Can you work these out from the model? Positions are in its coordinate system, mm. Face numbers are marked on the shaded views. A direction names the side the tool comes from. Round coordinates to 2 decimals unless told otherwise and drop trailing zeros. Write each loop counter-clockwise with the first axis right and the second up, starting at its lowest first coordinate (ties: lowest second). Pieces come first, ordered by that corner, then holes. Notation, with made-up numbers: M -9,6.25 L 40,6.25 A25 ccw 40,44.25 Z; hole C 9.25,-25 d1. An arc over 180 degrees is marked long. Use one line per item in the form item = value. Start each with the question number.
```python
from build123d import *

# Parameters (mm, degrees)
SKETCH1_W           = 20.1
SKETCH1_H           = 20.1
BOSS_EXTRUDE1_DEPTH = 40
SKETCH1_3_R         = 5.1
BOSS_EXTRUDE2_DEPTH = 10
SKETCH1_4_R         = 13
SKETCH1_4_R_2       = 2.1
BOSS_EXTRUDE3_DEPTH = 3
SKETCH2_R           = 5.05
CUT_EXTRUDE1_DEPTH  = 62
SKETCH2_3_R         = 5.05
SKETCH2_3_R_2       = 2.6
BOSS_EXTRUDE5_DEPTH = 26.5
SKETCH2_4_R         = 5.05
SKETCH2_4_R_2       = 2.6
CUT_EXTRUDE2_DEPTH  = 23.3
SKETCH2_5_R         = 5.05
SKETCH2_5_R_2       = 2.6
BOSS_EXTRUDE6_DEPTH = 3.2
CUT_EXTRUDE3_START  = 127.2
SKETCH2_6_R         = 5.05
CUT_EXTRUDE3_DEPTH  = 127.2
BOSS_EXTRUDE7_START = 100
SKETCH2_7_R         = 5.05
SKETCH2_7_R_2       = 2.6
BOSS_EXTRUDE7_DEPTH = 100
CUT_EXTRUDE4_START  = 96.8
SKETCH2_8_R         = 5.05
SKETCH2_8_R_2       = 2.6
CUT_EXTRUDE4_DEPTH  = 96.8
BOSS_EXTRUDE8_START = 76.7
SKETCH2_9_R         = 5.05
SKETCH2_9_R_2       = 2.6
BOSS_EXTRUDE8_DEPTH = 76.7
CUT_EXTRUDE5_START  = 73.5
SKETCH2_10_R        = 5.05
SKETCH2_10_R_2      = 2.6
CUT_EXTRUDE5_DEPTH  = 73.5
SKETCH3_W           = 73.5
SKETCH3_H           = 30
CUT_EXTRUDE6_DEPTH  = 10
FILLET1_R           = 3


with BuildPart() as part:
    # Sketch1 → Boss-Extrude1 (new body)
    with BuildSketch(Plane(origin=(0, 0, 0), x_dir=(1, 0, 0), z_dir=(0, 1, 0))):
        with BuildLine():
            Line((-160, 14.285714286), (-160, -114.285714286))
            ThreePointArc((-160, -114.285714286), (-70, -125.097415446), (20, -114.285714286))
            ThreePointArc((20, -114.285714286), (29.379159313, -50), (20, 14.285714286))
            ThreePointArc((20, 14.285714286), (-70, 25.097415446), (-160, 14.285714286))
        make_face()
        with Locations((-140, 0)):
            Rectangle(SKETCH1_W, SKETCH1_H, mode=Mode.SUBTRACT)
        Rectangle(SKETCH1_W, SKETCH1_H, mode=Mode.SUBTRACT)
        with Locations((-140, -100)):
            Rectangle(SKETCH1_W, SKETCH1_H, mode=Mode.SUBTRACT)
        with Locations((0, -100)):
            Rectangle(SKETCH1_W, SKETCH1_H, mode=Mode.SUBTRACT)
        Polygon((-126.75, 10.05), (-126.75, -13.25), (-150.05, -13.25), (-150.05, -86.75), (-126.75, -86.75), (-126.75, -110.05), (-13.25, -110.05), (-13.25, -86.75), (10.05, -86.75), (10.05, -13.25), (-13.25, -13.25), (-13.25, 10.05), align=None, mode=Mode.SUBTRACT)
    extrude(amount=BOSS_EXTRUDE1_DEPTH)

    # Sketch1<3> → Boss-Extrude2 (add)
    with BuildSketch(Plane(origin=(0, 0, 0), x_dir=(1, 0, 0), z_dir=(0, 1, 0))):
        Polygon((-13.25, 10.05), (-126.75, 10.05), (-126.75, -13.25), (-150.05, -13.25), (-150.05, -86.75), (-126.75, -86.75), (-126.75, -110.05), (-13.25, -110.05), (-13.25, -86.75), (10.05, -86.75), (10.05, -13.25), (-13.25, -13.25), align=None)
        with Locations(Location((-120, -50, 0), (0, 0, 270))):
            Circle(SKETCH1_3_R, mode=Mode.SUBTRACT)
        with BuildLine():
            ThreePointArc((-93.167984839, -59.230769231), (-90.236760582, -50), (-93.167984839, -40.769230769))
            ThreePointArc((-93.167984839, -40.769230769), (-92.071067812, -27.928932188), (-79.230769231, -26.832015161))
            ThreePointArc((-79.230769231, -26.832015161), (-70, -29.763239418), (-60.769230769, -26.832015161))
            ThreePointArc((-60.769230769, -26.832015161), (-47.928932188, -27.928932188), (-46.832015161, -40.769230769))
            ThreePointArc((-46.832015161, -40.769230769), (-49.763239418, -50), (-46.832015161, -59.230769231))
            ThreePointArc((-46.832015161, -59.230769231), (-47.928932188, -72.071067812), (-60.769230769, -73.167984839))
            ThreePointArc((-60.769230769, -73.167984839), (-70, -70.236760582), (-79.230769231, -73.167984839))
            ThreePointArc((-79.230769231, -73.167984839), (-92.071067812, -72.071067812), (-93.167984839, -59.230769231))
        make_face(mode=Mode.SUBTRACT)
        with Locations(Location((-35, -89.95, 0), (0, 0, 270))):
            Circle(SKETCH1_3_R, mode=Mode.SUBTRACT)
        with Locations(Location((-35, -10.05, 0), (0, 0, 270))):
            Circle(SKETCH1_3_R, mode=Mode.SUBTRACT)
    extrude(amount=BOSS_EXTRUDE2_DEPTH)

    # Sketch1<4> → Boss-Extrude3 (add)
    with BuildSketch(Plane(origin=(0, 0, 0), x_dir=(1, 0, 0), z_dir=(0, 1, 0))):
        with BuildLine():
            ThreePointArc((-60.769230769, -73.167984839), (-70, -70.236760582), (-79.230769231, -73.167984839))
            ThreePointArc((-79.230769231, -73.167984839), (-92.071067812, -72.071067812), (-93.167984839, -59.230769231))
            ThreePointArc((-93.167984839, -59.230769231), (-90.236760582, -50), (-93.167984839, -40.769230769))
            ThreePointArc((-93.167984839, -40.769230769), (-92.071067812, -27.928932188), (-79.230769231, -26.832015161))
            ThreePointArc((-79.230769231, -26.832015161), (-70, -29.763239418), (-60.769230769, -26.832015161))
            ThreePointArc((-60.769230769, -26.832015161), (-47.928932188, -27.928932188), (-46.832015161, -40.769230769))
            ThreePointArc((-46.832015161, -40.769230769), (-49.763239418, -50), (-46.832015161, -59.230769231))
            ThreePointArc((-46.832015161, -59.230769231), (-47.928932188, -72.071067812), (-60.769230769, -73.167984839))
        make_face()
        with Locations(Location((-70, -50, 0), (0, 0, 270))):
            Circle(SKETCH1_4_R, mode=Mode.SUBTRACT)
        with Locations(Location((-85, -65, 0), (0, 0, 270))):
            Circle(SKETCH1_4_R_2, mode=Mode.SUBTRACT)
        with Locations(Location((-55, -65, 0), (0, 0, 270))):
            Circle(SKETCH1_4_R_2, mode=Mode.SUBTRACT)
        with Locations(Location((-55, -35, 0), (0, 0, 270))):
            Circle(SKETCH1_4_R_2, mode=Mode.SUBTRACT)
        with Locations(Location((-85, -35, 0), (0, 0, 270))):
            Circle(SKETCH1_4_R_2, mode=Mode.SUBTRACT)
    extrude(amount=BOSS_EXTRUDE3_DEPTH)

    # Sketch2 → Cut-Extrude1 (cut)
    with BuildSketch(Plane.XY.offset(13.25)):
        with Locations((0, 25)):
            Circle(SKETCH2_R)
        with Locations((-140, 25)):
            Circle(SKETCH2_R)
    extrude(amount=-CUT_EXTRUDE1_DEPTH, mode=Mode.SUBTRACT)

    # Sketch2<3> → Boss-Extrude5 (add)
    # profile 1 of 2: a face of its own
    with BuildSketch(Plane.XY.offset(13.25)):
        with Locations((0, 25)):
            Circle(SKETCH2_3_R)
        with Locations((0, 25)):
            Circle(SKETCH2_3_R_2, mode=Mode.SUBTRACT)
    # profile 2 of 2: a face of its own
    with BuildSketch(Plane.XY.offset(13.25)):
        with Locations((-140, 25)):
            Circle(SKETCH2_3_R)
        with Locations((-140, 25)):
            Circle(SKETCH2_3_R_2, mode=Mode.SUBTRACT)
    extrude(amount=-BOSS_EXTRUDE5_DEPTH)

    # Sketch2<4> → Cut-Extrude2 (cut)
    # profile 1 of 2: a face of its own
    with BuildSketch(Plane.XY.offset(13.25)):
        with Locations((0, 25)):
            Circle(SKETCH2_4_R)
        with Locations((0, 25)):
            Circle(SKETCH2_4_R_2, mode=Mode.SUBTRACT)
    # profile 2 of 2: a face of its own
    with BuildSketch(Plane.XY.offset(13.25)):
        with Locations((-140, 25)):
            Circle(SKETCH2_4_R)
        with Locations((-140, 25)):
            Circle(SKETCH2_4_R_2, mode=Mode.SUBTRACT)
    extrude(amount=-CUT_EXTRUDE2_DEPTH, mode=Mode.SUBTRACT)

    # Sketch2<5> → Boss-Extrude6 (add)
    # profile 1 of 2: a face of its own
    with BuildSketch(Plane.XY.offset(13.25)):
        with Locations((0, 25)):
            Circle(SKETCH2_5_R)
        with Locations((0, 25)):
            Circle(SKETCH2_5_R_2, mode=Mode.SUBTRACT)
    # profile 2 of 2: a face of its own
    with BuildSketch(Plane.XY.offset(13.25)):
        with Locations((-140, 25)):
            Circle(SKETCH2_5_R)
        with Locations((-140, 25)):
            Circle(SKETCH2_5_R_2, mode=Mode.SUBTRACT)
    extrude(amount=-BOSS_EXTRUDE6_DEPTH)

    # Sketch2<6> → Cut-Extrude3 (cut)
    with BuildSketch(Plane.XY.offset(13.25).offset(CUT_EXTRUDE3_START)):
        with Locations((0, 25)):
            Circle(SKETCH2_6_R)
        with Locations((-140, 25)):
            Circle(SKETCH2_6_R)
    extrude(amount=-CUT_EXTRUDE3_DEPTH, mode=Mode.SUBTRACT)

    # Sketch2<7> → Boss-Extrude7 (add)
    # profile 1 of 2: a face of its own
    with BuildSketch(Plane.XY.offset(13.25).offset(BOSS_EXTRUDE7_START)):
        with Locations((0, 25)):
            Circle(SKETCH2_7_R)
        with Locations((0, 25)):
            Circle(SKETCH2_7_R_2, mode=Mode.SUBTRACT)
    # profile 2 of 2: a face of its own
    with BuildSketch(Plane.XY.offset(13.25).offset(BOSS_EXTRUDE7_START)):
        with Locations((-140, 25)):
            Circle(SKETCH2_7_R)
        with Locations((-140, 25)):
            Circle(SKETCH2_7_R_2, mode=Mode.SUBTRACT)
    extrude(amount=-BOSS_EXTRUDE7_DEPTH)

    # Sketch2<8> → Cut-Extrude4 (cut)
    # profile 1 of 2: a face of its own
    with BuildSketch(Plane.XY.offset(13.25).offset(CUT_EXTRUDE4_START)):
        with Locations((0, 25)):
            Circle(SKETCH2_8_R)
        with Locations((0, 25)):
            Circle(SKETCH2_8_R_2, mode=Mode.SUBTRACT)
    # profile 2 of 2: a face of its own
    with BuildSketch(Plane.XY.offset(13.25).offset(CUT_EXTRUDE4_START)):
        with Locations((-140, 25)):
            Circle(SKETCH2_8_R)
        with Locations((-140, 25)):
            Circle(SKETCH2_8_R_2, mode=Mode.SUBTRACT)
    extrude(amount=-CUT_EXTRUDE4_DEPTH, mode=Mode.SUBTRACT)

    # Sketch2<9> → Boss-Extrude8 (add)
    # profile 1 of 2: a face of its own
    with BuildSketch(Plane.XY.offset(13.25).offset(BOSS_EXTRUDE8_START)):
        with Locations((0, 25)):
            Circle(SKETCH2_9_R)
        with Locations(Location((0, 25, 0), (0, 0, 180))):
            Circle(SKETCH2_9_R_2, mode=Mode.SUBTRACT)
    # profile 2 of 2: a face of its own
    with BuildSketch(Plane.XY.offset(13.25).offset(BOSS_EXTRUDE8_START)):
        with Locations((-140, 25)):
            Circle(SKETCH2_9_R)
        with Locations(Location((-140, 25, 0), (0, 0, 180))):
            Circle(SKETCH2_9_R_2, mode=Mode.SUBTRACT)
    extrude(amount=-BOSS_EXTRUDE8_DEPTH)

    # Sketch2<10> → Cut-Extrude5 (cut)
    # profile 1 of 4: a face of its own
    with BuildSketch(Plane.XY.offset(13.25).offset(CUT_EXTRUDE5_START)):
        with Locations((-140, 25)):
            Circle(SKETCH2_10_R)
        with Locations((-140, 25)):
            Circle(SKETCH2_10_R_2, mode=Mode.SUBTRACT)
    # profile 2 of 4: a face of its own
    with BuildSketch(Plane.XY.offset(13.25).offset(CUT_EXTRUDE5_START)):
        with Locations((-140, 25)):
            Circle(SKETCH2_10_R_2)
    # profile 3 of 4: a face of its own
    with BuildSketch(Plane.XY.offset(13.25).offset(CUT_EXTRUDE5_START)):
        with Locations((0, 25)):
            Circle(SKETCH2_10_R)
        with Locations((0, 25)):
            Circle(SKETCH2_10_R_2, mode=Mode.SUBTRACT)
    # profile 4 of 4: a face of its own
    with BuildSketch(Plane.XY.offset(13.25).offset(CUT_EXTRUDE5_START)):
        with Locations((0, 25)):
            Circle(SKETCH2_10_R_2)
    extrude(amount=-CUT_EXTRUDE5_DEPTH, mode=Mode.SUBTRACT)

    # Sketch3 → Cut-Extrude6 (cut)
    with BuildSketch(Plane(origin=(-150.05, 0, 0), x_dir=(0, 0, -1), z_dir=(1, 0, 0))):
        with Locations((-50, 25)):
            Rectangle(SKETCH3_W, SKETCH3_H)
    extrude(amount=-CUT_EXTRUDE6_DEPTH, mode=Mode.SUBTRACT)

    # Fillet1
    fillet1_edges = [part.edges().sort_by_distance(p)[0] for p in [
        (10.05, 10, 50),
        (-1.6, 10, 13.25),
        (-13.25, 10, 1.6),
        (-70, 10, -10.05),
        (-143.375, 10, 13.25),
        (-143.375, 10, 86.75),
        (-126.75, 10, 98.4),
        (-70, 10, 110.05),
        (-13.25, 10, 98.4),
        (-1.6, 10, 86.75),
        (-126.75, 10, 1.6),
        (-126.75, 25, 86.75),
        (-126.75, 25, 110.05),
        (-13.25, 25, 110.05),
        (-13.25, 25, 86.75),
        (10.05, 25, 86.75),
        (10.05, 25, 13.25),
        (-13.25, 25, 13.25),
        (-13.25, 25, -10.05),
        (-126.75, 25, -10.05),
        (-126.75, 25, 13.25),
        (20, 20, 114.285714286),
        (-160, 20, 114.285714286),
        (-160, 20, -14.285714286),
        (20, 20, -14.285714286),
    ]]
    fillet(fillet1_edges, radius=FILLET1_R)


solid = part.part
```
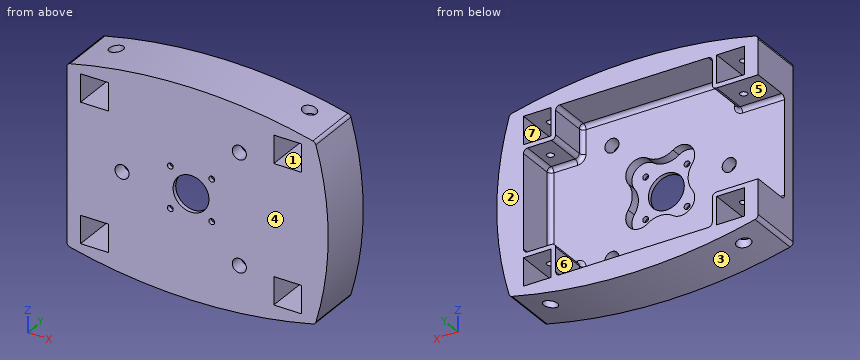
1. Please list where these lines run through material, in increasing order: line 1 along X through (y, z) = (1.5, 50); line 2 along Z through (x, y) = (-136.5, 25.5); line 3 along Y through (x, z) = (0, 111.95).
2. Will these pins go through, and if not, where does the flat tip stop? pin 1 (1 mm diameter, centred on x = -2, y = 12, fed in from +Z); pin 2 (8 mm diameter, centred on x = 0, y = 27, fed in from -Z); pin 3 (4 mm diameter, centred on x = -84.5, z = 84, fed in from +Y); pin 4 (9 mm diameter, centred on x = -35, z = 89.95, fed in from +Y).
3. If we section it at A-A (x = -70): List the corners of the cut face in (y, z) for me, and give its area (3 significant figures).
4. Which directions (+Z, -Z, +X, -X, +Y, -Y) give clear straight access to the entire face, cutting with the end or side of a thin tool? Please do the marked faces 4, 5, 6 and 7.
5. If we section it at B-B (z = 50): List the corners of the cut face in (x, y) for me.
6. If we mould it in two halves opening along Z, with no side actions, what happens to the marked faces 1, 2 and 3? For each: pulls with the +Z half, pulls with the -Z half, needs draft (parallel to the pull), parting line crosses it, or undercut.
7. If we section it at D-D (z = 99): List the corners of the cut face in (x, y) for me, and give its area (3 significant figures).
8. If we section it at C-C (x = -35): List the corners of the cut face in (y, z) for me.
Model answer:
q1.line_1 = -160 to -125.1, -114.9 to -83, -57 to 29.38
q1.line_2 = -13.25 to -10.05, 10.05 to 13.25, 86.75 to 89.95, 110.05 to 113.25
q1.line_3 = 0 to 22.4, 27.6 to 40
q2.pin_1 = 119.05
q2.pin_2 = -19.28
q2.pin_3 = 10
q2.pin_4 = through
q3.outline = M 0,-25.1 L 40,-25.1 L 40,-10.05 L 13,-10.05 A3 cw 10,-7.05 L 10,29.76 L 3,29.76 L 3,37 L 0,37 Z; M 0,63 L 3,63 L 3,70.24 L 10,70.24 L 10,107.05 A3 cw 13,110.05 L 40,110.05 L 40,125.1 L 0,125.1 Z
q3.area = 2,050 mm2
q4.face_4 = +Z, -Z, +X, -X, -Y
q4.face_5 = -X, +Y
q4.face_6 = +Y
q4.face_7 = +Y, -Y
q5.outline = M -160,0 L -125.1,0 L -125.1,10 L -160,10 Z; M -114.9,0 L -83,0 L -83,3 L -90.24,3 L -90.24,10 L -114.9,10 Z; M -57,0 L 29.38,0 L 29.38,40 L 10.05,40 L 10.05,13 A3 cw 7.05,10 L -49.76,10 L -49.76,3 L -57,3 Z
q6.face_1 = undercut
q6.face_2 = needs draft
q6.face_3 = pulls with the -Z half
q7.outline = M -160,0 L -150.05,0 L -150.05,40 L -160,40 Z; M -129.95,0 L -10.05,0 L -10.05,40 L -13.25,40 L -13.25,13 A3 cw -16.25,10 L -123.75,10 A3 cw -126.75,13 L -126.75,40 L -129.95,40 Z; M 10.05,0 L 23.98,0 L 23.98,40 L 10.05,40 Z
q7.area = 2,350 mm2
q8.outline = M 0,-23.48 L 40,-23.48 L 40,-10.05 L 13,-10.05 A3 cw 10,-7.05 L 10,4.95 L 0,4.95 Z; M 0,15.15 L 10,15.15 L 10,84.85 L 0,84.85 Z; M 0,95.05 L 10,95.05 L 10,107.05 A3 cw 13,110.05 L 40,110.05 L 40,123.48 L 0,123.48 Z
